from build123d import *

# Parameters (mm, degrees)
CROQUIS7_R                 = 40
SALIENTE_EXTRUIR3_DEPTH    = 60
CORTAR_EXTRUIR2_DEPTH      = 83.462112512
CORTAR_EXTRUIR2_DEPTH_BACK = 83.462112512
CROQUIS8_W                 = 6.5
CROQUIS8_H                 = 41
CROQUIS9_W                 = 4
CROQUIS9_H                 = 1.5
CORTAR_EXTRUIR3_DEPTH      = 43
CROQUIS11_R                = 34
CORTAR_EXTRUIR4_DEPTH      = 1
CROQUIS12_R                = 9.5
CORTAR_EXTRUIR5_DEPTH      = 110
CORTAR_EXTRUIR6_DEPTH      = 83.462112512
CORTAR_EXTRUIR6_DEPTH_BACK = 83.462112512
CROQUIS13_R                = 60.833333333
CROQUIS14_R                = 9.5
SALIENTE_EXTRUIR4_DEPTH    = 15
REDONDEO1_R                = 1
CROQUIS15_R                = 10.5
CROQUIS15_R_2              = 9.5
CORTAR_EXTRUIR7_DEPTH      = 0.5


# Read off the part's stored shape, not the designer's step: Simetría6
with BuildPart() as part:
    # Croquis7 → Saliente-Extruir3 (new body)
    with BuildSketch(Plane(origin=(0, 0, 0), x_dir=(1, 0, 0), z_dir=(0, 1, 0))):
        with Locations(Location((0, 0, 0), (0, 0, 270))):
            Circle(CROQUIS7_R)
    extrude(amount=-SALIENTE_EXTRUIR3_DEPTH)

    # Croquis8 → Cortar-Extruir2 (cut, two sides: drawn at the far end of the back side and taken through both)
    with BuildSketch(Plane(origin=(0, 0, 0), x_dir=(0, 0, -1), z_dir=(1, 0, 0)).offset(-CORTAR_EXTRUIR2_DEPTH_BACK)):
        with Locations((36.75, -39.5)):
            Rectangle(CROQUIS8_W, CROQUIS8_H)
        with Locations((-36.75, -39.5)):
            Rectangle(CROQUIS8_W, CROQUIS8_H)
    extrude(amount=CORTAR_EXTRUIR2_DEPTH + CORTAR_EXTRUIR2_DEPTH_BACK, mode=Mode.SUBTRACT)

    # Cortar-Barrer2: sweep along a curve in space
    with BuildLine() as cortar_barrer2_path:
        ThreePointArc((0, 0, 40), (28.284271247, 0, 28.284271247), (40, 0, 0))
        ThreePointArc((40, 0, 0), (28.284271247, 0, -28.284271247), (0, 0, -40))
        ThreePointArc((0, 0, -40), (-28.284271247, 0, -28.284271247), (-40, 0, 0))
        ThreePointArc((-40, 0, 0), (-28.284271247, 0, 28.284271247), (0, 0, 40))
    # Croquis9 → Cortar-Barrer2 (sweep, cut)
    with BuildSketch(Plane(origin=(0, 0, 0), x_dir=(0, 0, -1), z_dir=(1, 0, 0))):
        with Locations((-40, -6.75)):
            Rectangle(CROQUIS9_W, CROQUIS9_H)
        with Locations((-40, -11.25)):
            Rectangle(CROQUIS9_W, CROQUIS9_H)
        with Locations((-40, -15.75)):
            Rectangle(CROQUIS9_W, CROQUIS9_H)
    sweep(path=cortar_barrer2_path.line, mode=Mode.SUBTRACT)

    # Croquis10 → Cortar-Extruir3 (cut)
    with BuildSketch(Plane.XZ.offset(60)):
        with BuildLine():
            Line((-20.316249654, -28.5), (20.316249654, -28.5))
            ThreePointArc((20.316249654, -28.5), (35, 0), (20.316249654, 28.5))
            Line((20.316249654, 28.5), (-20.316249654, 28.5))
            ThreePointArc((-20.316249654, 28.5), (-35, 0), (-20.316249654, -28.5))
        make_face()
    extrude(amount=-CORTAR_EXTRUIR3_DEPTH, mode=Mode.SUBTRACT)

    # Croquis11 → Cortar-Extruir4 (cut)
    with BuildSketch(Plane(origin=(0, 0, 0), x_dir=(1, 0, 0), z_dir=(0, 1, 0))):
        with Locations(Location((0, 0, 0), (0, 0, 270))):
            Circle(CROQUIS11_R)
    extrude(amount=-CORTAR_EXTRUIR4_DEPTH, mode=Mode.SUBTRACT)

    # Croquis12 → Cortar-Extruir5 (cut)
    with BuildSketch(Plane.XY.offset(33.5)):
        with Locations((0, -30.5)):
            Circle(CROQUIS12_R)
    extrude(amount=-CORTAR_EXTRUIR5_DEPTH, mode=Mode.SUBTRACT)

    # Croquis13 → Cortar-Extruir6 (cut, two sides: drawn at the far end of the back side and taken through both)
    with BuildSketch(Plane.XY.offset(-CORTAR_EXTRUIR6_DEPTH_BACK)):
        with Locations((0, -105.833333333)):
            Circle(CROQUIS13_R)
    extrude(amount=CORTAR_EXTRUIR6_DEPTH + CORTAR_EXTRUIR6_DEPTH_BACK, mode=Mode.SUBTRACT)

    # Croquis14 → Saliente-Extruir4 (add)
    with BuildSketch(Plane(origin=(0, 0, 28.5), x_dir=(-1, 0, 0), z_dir=(0, 0, -1))):
        with BuildLine():
            Line((-12.5, -30.5), (-12.5, -17))
            Line((-12.5, -17), (12.5, -17))
            Line((12.5, -17), (12.5, -30.5))
            ThreePointArc((12.5, -30.5), (0, -43), (-12.5, -30.5))
        make_face()
        with Locations(Location((0, -30.5, 0), (0, 0, 180))):
            Circle(CROQUIS14_R, mode=Mode.SUBTRACT)
    saliente_extruir4 = extrude(amount=SALIENTE_EXTRUIR4_DEPTH)

    # Redondeo1
    redondeo1_edges = [part.edges().sort_by_distance(p)[0] for p in [
        (0, -43, 28.5),
        (-12.5, -23.75, 28.5),
        (12.5, -23.75, 28.5),
    ]]
    fillet(redondeo1_edges, radius=REDONDEO1_R)

    # Simetría4: Saliente-Extruir4 across plane
    add(saliente_extruir4.mirror(Plane.XY))

    # Simetría6
    split(bisect_by=Plane.XY, keep=Keep.TOP)

    # Simetr_a6 2: part across plane


with BuildPart() as part_1:
    add(part.part)
    add(part.part.mirror(Plane.XY))

    # Croquis15 → Cortar-Extruir7 (cut, symmetric)
    with BuildSketch(Plane(origin=(0, 0, -31.5), x_dir=(-1, 0, 0), z_dir=(0, 0, -1))):
        with Locations((0, -30.5)):
            Circle(CROQUIS15_R)
        with Locations((0, -30.5)):
            Circle(CROQUIS15_R_2, mode=Mode.SUBTRACT)
    cortar_extruir7 = extrude(amount=CORTAR_EXTRUIR7_DEPTH, both=True, mode=Mode.SUBTRACT)

    # Simetría7: Cortar-Extruir7 across plane
    add(cortar_extruir7.mirror(Plane.XY), mode=Mode.SUBTRACT)


solid = part_1.part
CAD build for the part. Positions are in the model's coordinates, mm. A direction names the side the tool comes from. Coordinates: 2 decimals unless noted, no trailing zeros. Loops run counter-clockwise (first coordinate to the right, second up) from the corner with the lowest first, then second, coordinate; pieces in that order, holes last. Notation, with made-up numbers: (6.25, 44.25) -> (45.25, 44.25) arc R13 cw to (45.25, 67.25) -> close; hole circle Ø11 at (43.25, -14.75). An arc over 180 degrees is marked (long way). One line per item, written item: value.
1. Drill centre lines: line 1 (Z direction, x = -11.5, y = -41.5); line 2 (X direction, y = -30, z = 19); line 3 (X direction, y = -30.5, z = 18.5). Where is each one in solid material? Low to high. Write a range as [from, to].
Answers:
line 1: z = [-33.5, -28.5], [28.5, 33.5]
line 2: x = [-35.2, -29.39], [-12.5, -9.49], [9.49, 12.5], [29.39, 35.2]
line 3: x = [-35.46, -29.71], [-12.5, -9.5], [9.5, 12.5], [29.71, 35.46]
2. Pull direction Y, two halves, no side cores. Call faces 4 (the face through (-3, -21, -13.5)), 5 (the face through (0, -19, -36)), 6 (the face through (1.37, -20.09, -31.51)): pulls with the +Y half, pulls with the -Y half, needs draft (parallel to the pull), parting line crosses it, or undercut.
Answers:
face 4: needs draft
face 5: pulls with the -Y half
face 6: undercut
3. Which spindle directions (+Z, -Z, +X, -X, +Y, -Y) get a long thin tool onto all of the face, cutting with end or side? Do faces 1 (the face through (0, -41, -33.5)), 2 (the face through (35.4, -15, -14.7)), 3 (the face through (4.8, -43.5, -28.5)). Say none if no direction does.
Answers:
face 1: -Z, +X, -X, -Y
face 2: none
face 3: -Y
4. Slice it at A-A on y = -46.5. Write the cut outline in (x, z).
Answers:
outline: (-21.86, -33.5) -> (-13.43, -33.5) -> (-13.43, -28.5) -> (-20.32, -28.5) arc R35 cw to (-20.32, 28.5) -> (-13.43, 28.5) -> (-13.43, 33.5) -> (-21.86, 33.5) arc R40 ccw to start; (13.43, -33.5) -> (21.86, -33.5) arc R40 ccw to (21.86, 33.5) -> (13.43, 33.5) -> (13.43, 28.5) -> (20.32, 28.5) arc R35 cw to (20.32, -28.5) -> (13.43, -28.5) -> close
5. Slice it at B-B on x = -8. Give the number of separate pieces and of enclosed holes in the cut face, and give its area (3 significant figures).
Answers:
separate pieces: 3
enclosed holes: 0
area: 1,830 mm^2
6. Flat gauge pins, fed straight in: P1, Ø12, axis at x = -20, z = -9.5, coming from the -Y side; P2, Ø12, axis at y = -32, z = -9, coming from the -X side; P3, Ø11, axis at y = -24.5, z = -19, coming from the +X side. Where does each tip first touch, or does it go through?
Answers:
P1: stops at y = -17
P2: stops at x = -39.89
P3: stops at x = 37.65
